Part model, mm, in its own coordinate system. Face numbers are marked on the shaded views. Give positions to 0.01 mm unless a question says otherwise; leave off trailing zeros. Order: outer loops, then holes, each group sorted by start corner. A loop starts at its lowest first (then second) coordinate and runs counter-clockwise, first axis right, second up.
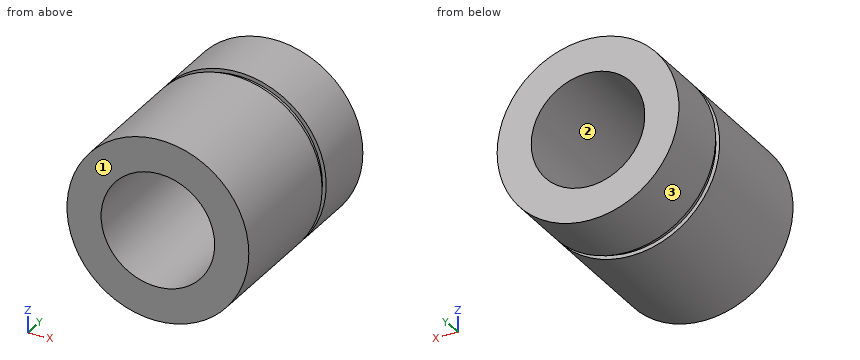
from build123d import *

# Parameters (mm, degrees)
SKIZZE1_R                       = 12
SKIZZE1_R_2                     = 7.5
AUFSATZ_LINEAR_AUSTRAGEN1_DEPTH = 28
SCHNITT_LINEAR_START            = 9
SKIZZE2_R                       = 12
SKIZZE2_R_2                     = 11.5
SCHNITT_LINEAR_AUSTRAGEN1_DEPTH = 1


with BuildPart() as part:
    # Skizze1 → Aufsatz-Linear austragen1 (new body)
    with BuildSketch(Plane(origin=(0, 0, 0), x_dir=(1, 0, 0), z_dir=(0, 1, 0))):
        Circle(SKIZZE1_R)
        Circle(SKIZZE1_R_2, mode=Mode.SUBTRACT)
    extrude(amount=AUFSATZ_LINEAR_AUSTRAGEN1_DEPTH)

    # Skizze2 → Schnitt-Linear austragen1 (cut)
    with BuildSketch(Plane.XZ.offset(-28).offset(SCHNITT_LINEAR_START)):
        Circle(SKIZZE2_R)
        Circle(SKIZZE2_R_2, mode=Mode.SUBTRACT)
    extrude(amount=SCHNITT_LINEAR_AUSTRAGEN1_DEPTH, mode=Mode.SUBTRACT)


solid = part.part
Item 1: Band-saw the part on B-B on z = 0. List the corners of the cut face in (x, y).
Item 2: Drill centre lines: probe 1 along Z at (x, y) = (0, 12); probe 2 along Y at (x, z) = (-7.5, 9). Where is each one in solid material? Low to high.
Item 3: Band-saw the part on D-D on x = 8.5. List the corners of the cut face in (y, z).
Item 4: Band-saw the part on C-C on z = -8.25. List the corners of the cut face in (x, y).
Item 5: Drop flat-ended pins along their axis: P1, Ø1, axis at x = 8, y = 17, coming from the -Z side; P2, Ø2, axis at x = 0.5, y = 23.5, coming from the -Z side; P3, Ø3, axis at y = 23.5, z = -3.5, coming from the -X side; P4, Ø4, axis at y = 9, z = -2.5, coming from the +X side. Give the stop position or say it passes through.
Item 6: Pull direction X, two halves, no side cores. Call the marked faces 1, 2 and 3: released by +X, released by -X, zero draft, split by the parting line, or undercut.
Item 7: Band-saw the part on A-A on x = 0. List the corners of the cut face in (y, z).
Working result:
1. outline: (-12, 0) - (-7.5, 0) - (-7.5, 28) - (-12, 28) - (-12, 19) - (-11.5, 19) - (-11.5, 18) - (-12, 18) - close; (7.5, 0) - (12, 0) - (12, 18) - (11.5, 18) - (11.5, 19) - (12, 19) - (12, 28) - (7.5, 28) - close
2. probe 1: z = -12 to -7.5, 7.5 to 12
2. probe 2: y = 0 to 18, 19 to 28
3. outline: (0, -8.47) - (18, -8.47) - (18, -7.75) - (19, -7.75) - (19, -8.47) - (28, -8.47) - (28, 8.47) - (19, 8.47) - (19, 7.75) - (18, 7.75) - (18, 8.47) - (0, 8.47) - close
4. outline: (-8.71, 0) - (8.71, 0) - (8.71, 18) - (8.01, 18) - (8.01, 19) - (8.71, 19) - (8.71, 28) - (-8.71, 28) - (-8.71, 19) - (-8.01, 19) - (-8.01, 18) - (-8.71, 18) - close
5. P1: stops at z = -9.37
5. P2: stops at z = -12
5. P3: stops at x = -11.83
5. P4: stops at x = 11.99
6. face 1: zero draft
6. face 2: undercut
6. face 3: split by the parting line
7. outline: (0, -12) - (18, -12) - (18, -11.5) - (19, -11.5) - (19, -12) - (28, -12) - (28, -7.5) - (0, -7.5) - close; (0, 7.5) - (28, 7.5) - (28, 12) - (19, 12) - (19, 11.5) - (18, 11.5) - (18, 12) - (0, 12) - close
